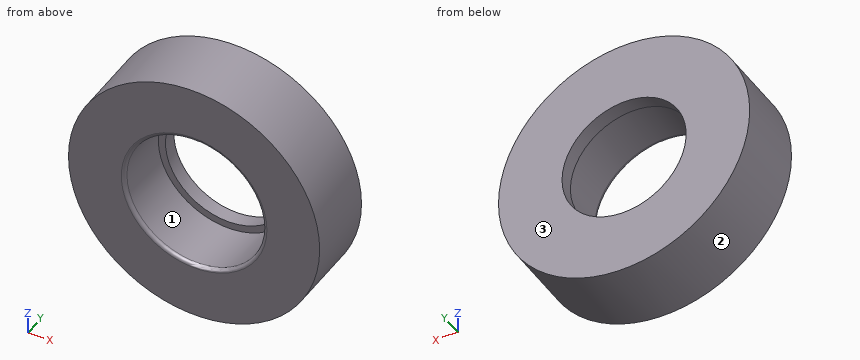
from build123d import *

# Parameters (mm, degrees)
SKETCH_1_R      = 17.5
SKETCH_1_R_2    = 9.65
EXTRUDE_1_DEPTH = 10
SKETCH_2_R      = 9.65
SKETCH_2_R_2    = 8.65
EXTRUDE_2_DEPTH = 2
FILLET_1_R      = 0.5


with BuildPart() as part:
    # Эскиз1 → Бобышка-Вытянуть1 (new body)
    with BuildSketch(Plane(origin=(0, 0, 0), x_dir=(1, 0, 0), z_dir=(0, 1, 0))):
        Circle(SKETCH_1_R)
        Circle(SKETCH_1_R_2, mode=Mode.SUBTRACT)
    extrude(amount=EXTRUDE_1_DEPTH)

    # Эскиз2 → Бобышка-Вытянуть2 (add)
    with BuildSketch(Plane(origin=(0, 10, 0), x_dir=(1, 0, 0), z_dir=(0, 1, 0))):
        Circle(SKETCH_2_R)
        Circle(SKETCH_2_R_2, mode=Mode.SUBTRACT)
    extrude(amount=-EXTRUDE_2_DEPTH)

    # Скругление1
    fillet_1_edges = [part.edges().sort_by_distance(p)[0] for p in [
        (-9.65, 0, 0),
    ]]
    fillet(fillet_1_edges, radius=FILLET_1_R)


solid = part.part
Geometry: final body of the model. Coordinates: model frame, mm. Face numbers are marked on the shaded views. Round coordinates to 2 decimals unless told otherwise and drop trailing zeros. Loops run counter-clockwise (first coordinate to the right, second up) from the corner with the lowest first, then second, coordinate; pieces in that order, holes last. Notation, with made-up numbers: M 61.5,-33.5 L 120.5,-33.5 A15 ccw 120.5,-18.5 Z; hole C 61,-26 d1. An arc over 180 degrees is marked long. Put each result on its own line as item: value. Start each with the question number.
(1) Section query A-A (z = 0). Return loops of the section in (x, y), then the cut area to 3 significant figures.
(2) Section query C-C (y = 8.5). Return loops of the section in (x, z), then the cut area to 3 significant figures.
(3) Contact query for flat-ended pins moving along their axis: pin 1 Ø3 at (y, z) = (5.5, 12) entering from -X; pin 2 Ø4 at (x, y) = (12, 4) entering from -Z; pin 3 Ø1.5 at (y, z) = (5.5, 7.5) entering from -X. Output: stop coordinate, or through.
(4) Draft query along Z for the marked faces 1, 2 and 3. Return one class per face: +Z half, -Z half, draft (parallel to the pull), parting line (faces both ways), or undercut.
(5) Section query B-B (y = 4). Return loops of the section in (x, z), then the cut area to 3 significant figures.
(6) Material intervals for line 1 along X through (y, z) = (9.2, 0); line 2 along X through (y, z) = (6, 0), sorted ascending. Write a range as [from, to].
(7) Section query D-D (x = 15.5). Return loops of the section in (y, z).
Findings below:
1. outline: M -17.5,0 L -10.15,0 A0.5 ccw -9.65,0.5 L -9.65,8 L -8.65,8 L -8.65,10 L -17.5,10 Z; M 8.65,8 L 9.65,8 L 9.65,0.5 A0.5 ccw 10.15,0 L 17.5,0 L 17.5,10 L 8.65,10 Z
1. area: 161 mm2
2. outline: C 0,0 d35; hole C 0,0 d17.3
2. area: 727 mm2
3. pin 1: stops at x = -14
3. pin 2: stops at z = -14.36
3. pin 3: stops at x = -16.15
4. face 1: undercut
4. face 2: parting line
4. face 3: draft
5. outline: C 0,0 d35; hole C 0,0 d19.3
5. area: 670 mm2
6. line 1: x = [-17.5, -8.65], [8.65, 17.5]
6. line 2: x = [-17.5, -9.65], [9.65, 17.5]
7. outline: M 0,-8.12 L 10,-8.12 L 10,8.12 L 0,8.12 Z
